Autodesk Inventor part; units mm, degrees
ref_plane "YZ Plane" through (0, 0, 0) normal (1, 0, 0) x (0, 1, 0)
ref_plane "XZ Plane" through (0, 0, 0) normal (0, 1, 0) x (-1, 0, 0)
ref_plane "XY Plane" through (0, 0, 0) normal (0, 0, 1) x (1, 0, 0)
sketch "Sketch1" plane through (0, 0, 0) normal (0, 0, 1) x (1, 0, 0)
  line L0 (-15.875, 0) -> (-12.7, 0)
  line L1 (-12.7, 0) -> (-12.7, 22.352)
  line L2 (-9.525, 25.527) -> (9.525, 25.527)
  line L3 (12.7, 22.352) -> (12.7, 0)
  line L4 (12.7, 0) -> (15.875, 0)
  line L5 (15.875, 0) -> (15.875, 25.527)
  line L6 (12.7, 28.702) -> (-12.7, 28.702)
  line L7 (-15.875, 25.527) -> (-15.875, 0)
  arc A0 (-9.525, 25.527) -> (-12.7, 22.352) centre (-9.525, 22.352) ccw
  arc A1 (12.7, 22.352) -> (9.525, 25.527) centre (9.525, 22.352) ccw
  arc A2 (-12.7, 28.702) -> (-15.875, 25.527) centre (-12.7, 25.527) ccw
  arc A3 (15.875, 25.527) -> (12.7, 28.702) centre (12.7, 25.527) ccw
  line L8 (0, 35.2315) -> (0, -5.8719)
  point P0 (0, 0)
  dimension "d0" = 28.702
  dimension "d1" = 31.75
  dimension "d2" = 3.175
  dimension "d3" = 3.175
  dimension "d4" = 3.175
extrude "Extrusion1" add sketch "Sketch1" along normal mid plane 76.2
sketch "Sketch4" plane through (15.875, 0, 38.1) normal (1, 0, 0) x (0, 0, -1)
  line L0 (-79.375, 0) -> (476.25, 0)
  line L1 (38.1, -5.7404) -> (38.1, 34.4424)
  circle A0 centre (38.1, 12.7) radius 3.175
  point P0 (38.1, 0)
  dimension "d35" = 12.7
  dimension "d36" = 0
  dimension "d37" = 6.35
extrude "Extrusion4" cut sketch "Sketch4" against normal up to surface (31.75 mm away)
pattern_linear "Rectangular Pattern3" count 20 spacing 25.4 along (0, 0, 1) count 20 spacing 25.4 along (0, 0, -1) of "Extrusion4"
equation "\"d5\" = SideLength"
equation "\"SideLength\" = 76.2"
properties part number "Electronics Board Raiser" material "Aluminum 6061"
The listing builds one solid part. Answer for the finished solid, in the listing's coordinates (mm). A direction names the side the tool comes from. Give positions to 0.01 mm unless a question says otherwise; leave off trailing zeros. Write each loop counter-clockwise with the first axis right and the second up, starting at its lowest first coordinate (ties: lowest second). Pieces come first, ordered by that corner, then holes. Notation, with made-up numbers: (-10, -7) - (-6, -7) arc R17 cw to (-6, 25) - close; hole circle Ø6 at (4.25, -30.75). An arc over 180 degrees is marked (long way). Use one line per item in the form item = value. Start each with the question number.
1) Find section B-B on y = 2.5. Determine the outline of the cut face in (x, z) (3 decimals).
2) Find section C-C on y = 12.7. Count the separate pieces of the cut face and the enclosed holes in it, plus the area to 3 significant figures.
3) Find section A-A on z = 25.4. Determine the outline of the cut face in (x, y) (3 decimals).
4) Flat-ended cylindrical pins translate along their axes: pin 1 Ø4 at (y, z) = (12.7, -25.4) entering from -X; pin 2 Ø3 at (x, z) = (-3, -26) entering from -Y; pin 3 Ø12 at (x, y) = (-11, 10) entering from +Z. Find the tip coordinate at first contact, or state that the pin passes through.
5) The mould has two halves that part along Y. Classify faces 1 (the face through (-14.97, 27.747, -0.533)), 2 (the face through (14.31, 11.48, -28.33)), 3 (the face through (11.745, 24.622, -0.533)): pulls with the +Y half, pulls with the -Y half, needs draft (parallel to the pull), parting line crosses it, or undercut.
6) A tool of negligible diameter and unlimited length cuts with its end or side. For faces 4 (the face through (12.7, 9, -1)), 5 (the face through (-15.875, 7, -1)), from which of +Z, -Z, +X, -X, +Y, -Y can it reach the whole face along a straight path? Write none if from no direction.
7) Find section D-D on z = -13. Determine the outline of the cut face in (x, y) (3 decimals).
8) Consider line 1 along Z through (x, y) = (14.5, 12.7) (3 decimals); line 2 along X through (y, z) = (10.5, 28.5) (3 decimals); line 3 along Y through (x, z) = (-0.5, -1.5). Determine where each line is inside the solid, lowest interval first. Write a range as from..to.
Geometry results:
q1.outline = (-15.875, -38.1) - (-12.7, -38.1) - (-12.7, 38.1) - (-15.875, 38.1) - close; (12.7, -38.1) - (15.875, -38.1) - (15.875, 38.1) - (12.7, 38.1) - close
q2.separate_pieces = 8
q2.enclosed_holes = 0
q2.area = 363 mm2
q3.outline = (-15.875, 0) - (-12.7, 0) - (-12.7, 9.525) - (-15.875, 9.525) - close; (-15.875, 15.875) - (-12.7, 15.875) - (-12.7, 22.352) arc R3.175 cw to (-9.525, 25.527) - (9.525, 25.527) arc R3.175 cw to (12.7, 22.352) - (12.7, 15.875) - (15.875, 15.875) - (15.875, 25.527) arc R3.175 ccw to (12.7, 28.702) - (-12.7, 28.702) arc R3.175 ccw to (-15.875, 25.527) - close; (12.7, 0) - (15.875, 0) - (15.875, 9.525) - (12.7, 9.525) - close
q4.pin_1 = through
q4.pin_2 = 25.53
q4.pin_3 = 38.1
q5.face_1 = pulls with the +Y half
q5.face_2 = undercut
q5.face_3 = pulls with the -Y half
q6.face_4 = +Z, -Z, -Y
q6.face_5 = +Z, -Z, -X, +Y, -Y
q7.outline = (-15.875, 0) - (-12.7, 0) - (-12.7, 22.352) arc R3.175 cw to (-9.525, 25.527) - (9.525, 25.527) arc R3.175 cw to (12.7, 22.352) - (12.7, 0) - (15.875, 0) - (15.875, 25.527) arc R3.175 ccw to (12.7, 28.702) - (-12.7, 28.702) arc R3.175 ccw to (-15.875, 25.527) - close
q8.line_1 = -38.1..-28.575, -22.225..-3.175, 3.175..22.225, 28.575..38.1
q8.line_2 = -15.875..-12.7, 12.7..15.875
q8.line_3 = 25.53..28.7
